```python
from build123d import *

# Parameters (mm, degrees)
SKETCH130_R     = 3.1
PAD039_DEPTH    = 20
POCKET048_DEPTH = 10
SKETCH131_R     = 4.6
POCKET047_DEPTH = 3


with BuildPart() as part:
    # Sketch130 → Pad039 (new body, symmetric)
    with BuildSketch(Plane.XZ):
        with BuildLine():
            Line((-64, 8), (11, 8))
            ThreePointArc((12, 7), (11.707107, 7.707107), (11, 8))
            Line((12, 7), (12, 0))
            ThreePointArc((9.499513, -5.362311), (11.344155, -2.958328), (12, 0))
            ThreePointArc((1.937819, -9.996123), (5.890842, -7.960183), (9.499513, -5.362311))
            ThreePointArc((-8.966462, -11.52862), (-3.413443, -11.48016), (1.937819, -9.996123))
            ThreePointArc((-17.077228, -2.032133), (-14.868336, -8.357429), (-8.966462, -11.52862))
            Line((-16.97253, 0.96604), (-17.077228, -2.032133))
            ThreePointArc((-16.97253, 0.96604), (-17.237697, 1.679846), (-17.928591, 2))
            Line((-17.928591, 2), (-64.086659, 4.001878))
            ThreePointArc((-64, 8), (-65.99953, 6.04334), (-64.086659, 4.001878))
        make_face()
        Circle(SKETCH130_R, mode=Mode.SUBTRACT)
    extrude(amount=PAD039_DEPTH, both=True)

    # Sketch133 → Pocket048 (cut)
    with BuildSketch(Plane.XZ.offset(20)):
        with BuildLine():
            Line((12, 6), (12, -34))
            Line((12, -34), (-17.928591, -34))
            Line((-17.928591, 2), (-17.928591, -34))
            ThreePointArc((0, 6.5), (-9.19194, 5.156963), (-17.928591, 2))
            ThreePointArc((12, 6), (6.010743, 6.507841), (0, 6.5))
        make_face()
    pocket048 = extrude(amount=-POCKET048_DEPTH, mode=Mode.SUBTRACT)

    # Sketch131 → Pocket047 (cut)
    with BuildSketch(Plane.XZ.offset(10)):
        Circle(SKETCH131_R)
    pocket047 = extrude(amount=-POCKET047_DEPTH, mode=Mode.SUBTRACT)

    # Mirrored009: Pocket047, Pocket048 across XZ
    add(pocket047.mirror(Plane.XZ), mode=Mode.SUBTRACT)
    add(pocket048.mirror(Plane.XZ), mode=Mode.SUBTRACT)


solid = part.part
```
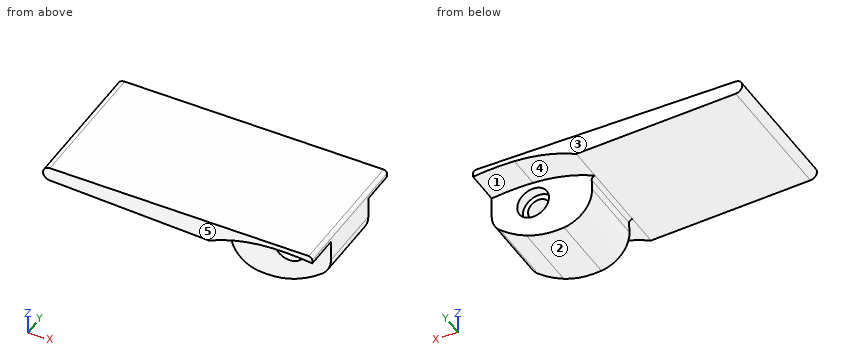
Here's how the part is built. I have some questions about the finished solid (model axes, mm). Face numbers are marked on the shaded views. A direction names the side the tool comes from. Give positions to 0.01 mm unless a question says otherwise; leave off trailing zeros. Order: outer loops, then holes, each group sorted by start corner. A loop starts at its lowest first (then second) coordinate and runs counter-clockwise, first axis right, second up. Notation, with made-up numbers: (49, 8.25) - (99, 8.25) arc R21 ccw to (99, 45.25) - close; hole circle Ø9 at (29, -30.5). An arc over 180 degrees is marked (long way). Answer as a JSON object with one key per item and string values. Group by question number.
Item 1: If we section it at B-B on y = 15: Please give me the cut outline in (x, z), and give its area (3 significant figures).
Item 2: If we section it at D-D on y = 9: Please give me the cut outline in (x, z), and give its area (3 significant figures).
Item 3: For P1, Ø1, axis at x = -50, y = -3.5, coming from the -Z side; P2, Ø8, axis at x = -3.5, z = -7, coming from the +Y side; P3, Ø10, axis at x = -0.5, z = 1, coming from the -Y side; P4, Ø5.5, axis at x = 0, z = 0, coming from the -Y side, each with a flat end and sliding along its axis, tell me the tip position at first contact or that it passes through.
Item 4: Which directions (+Z, -Z, +X, -X, +Y, -Y) give clear straight access to the entire face, cutting with the end or side of a thin tool? Please do the marked faces 4 and 5.
Item 5: If we section it at A-A on y = 4: Please give me the cut outline in (x, z).
Item 6: Please list where these lines run through material, in increasing order: probe 1 along Z at (x, y) = (0, 0.5); probe 2 along X at (y, z) = (9.5, -1.25); probe 3 along X at (y, z) = (-3.5, 0).
Item 7: If we mould it in two halves opening along X, with no side actions, what happens to the marked faces 1, 2 and 3? For each: pulls with the +X half, pulls with the -X half, needs draft (parallel to the pull), parting line crosses it, or undercut.
Item 8: If we section it at C-C on x = -10: Please give me the cut outline in (y, z).
Result set:
{
 "1": {"outline": "(-64.09, 4) - (-17.93, 2) arc R46.14 cw to (0, 6.5) arc R70 cw to (12, 6) - (12, 7) arc R1 ccw to (11, 8) - (-64, 8) arc R2 ccw to start", "area": "311 mm²"},
 "2": {"outline": "(-64.09, 4) - (-17.93, 2) arc R1 cw to (-16.97, 0.97) - (-17.08, -2.03) arc R9.24 ccw to (-8.97, -11.53) arc R21.27 ccw to (1.94, -10) arc R30 ccw to (9.5, -5.36) arc R7 ccw to (12, 0) - (12, 7) arc R1 ccw to (11, 8) - (-64, 8) arc R2 ccw to start; hole circle Ø9.2 at (0, 0)", "area": "676 mm²"},
 "3": {"P1": "z = 3.37", "P2": "y = 10", "P3": "y = -10", "P4": "through"},
 "4": {"face 4": "-Z, +Y", "face 5": "+Z, -Z, +X, -X, -Y"},
 "5": {"outline": "(-64.09, 4) - (-17.93, 2) arc R1 cw to (-16.97, 0.97) - (-17.08, -2.03) arc R9.24 ccw to (-8.97, -11.53) arc R21.27 ccw to (1.94, -10) arc R30 ccw to (9.5, -5.36) arc R7 ccw to (12, 0) - (12, 7) arc R1 ccw to (11, 8) - (-64, 8) arc R2 ccw to start; hole circle Ø6.2 at (0, 0)"},
 "6": {"probe 1": "-10.71 to -3.1, 3.1 to 8", "probe 2": "-17.05 to -4.43, 4.43 to 11.89", "probe 3": "-17.01 to -3.1, 3.1 to 12"},
 "7": {"face 1": "undercut", "face 2": "parting line crosses it", "face 3": "needs draft"},
 "8": {"outline": "(-20, 4.95) - (-10, 4.95) - (-10, -11.34) - (10, -11.34) - (10, 4.95) - (20, 4.95) - (20, 8) - (-20, 8) - close"}
}
